Source: CAD feature listing. Evaluate the final solid. Frame: model axes, mm. Face numbers are marked on the shaded views. A direction names the side the tool comes from. Give positions to 0.01 mm unless a question says otherwise; leave off trailing zeros. Loops run counter-clockwise (first coordinate to the right, second up) from the corner with the lowest first, then second, coordinate; pieces in that order, holes last.
from build123d import *

# Parameters (mm, degrees)
F0_R     = 317.5
F1_DEPTH = 127
F2_DEPTH = 177.8
F0_R_2   = 127
F3_DEPTH = 127
F4_R     = 152.4
F5_DEPTH = 127
F6_R     = 152.4
F7_DEPTH = 127


with BuildPart() as f1:
    # F0 (on Front) → F1 (new body)
    with BuildSketch(Plane.XZ):
        with BuildLine():
            ThreePointArc((2e-06, 508), (359.210245, 359.210244), (508, 0))
            ThreePointArc((508, 0), (359.210245, -359.210244), (2e-06, -508))
            Line((2e-06, -508), (1016, -508))
            Line((1016, -508), (1016, 508))
            Line((1016, 508), (2e-06, 508))
        make_face()
        with BuildLine():
            ThreePointArc((2e-06, -508), (-508, 0), (2e-06, 508))
            Line((2e-06, 508), (-1016, 508))
            Line((-1016, 508), (-1016, -508))
            Line((-1016, -508), (2e-06, -508))
        make_face()
        with BuildLine():
            ThreePointArc((2e-06, -508), (359.210245, -359.210244), (508, 0))
            ThreePointArc((508, 0), (359.210245, 359.210244), (2e-06, 508))
            ThreePointArc((2e-06, 508), (-508, 0), (2e-06, -508))
        make_face()
        Circle(F0_R, mode=Mode.SUBTRACT)
    extrude(amount=-F1_DEPTH)

    # F0 (on Front) → F2 (join)
    with BuildSketch(Plane.XZ):
        with BuildLine():
            ThreePointArc((2e-06, -508), (359.210245, -359.210244), (508, 0))
            ThreePointArc((508, 0), (359.210245, 359.210244), (2e-06, 508))
            ThreePointArc((2e-06, 508), (-508, 0), (2e-06, -508))
        make_face()
        Circle(F0_R, mode=Mode.SUBTRACT)
    extrude(amount=F2_DEPTH)

    # F0 (on Front) → F3 (join)
    with BuildSketch(Plane.XZ):
        Circle(F0_R)
        Circle(F0_R_2, mode=Mode.SUBTRACT)
    extrude(amount=-F3_DEPTH)

    # F4 (on face) → F5 (join)
    with BuildSketch(Plane(origin=(-1016, 0, 0), x_dir=(0, -1, 0), z_dir=(-1, 0, 0))):
        with BuildLine():
            Line((-127, -508), (-127, 508))
            Line((-127, 508), (-939.8, 508))
            ThreePointArc((-939.8, 508), (-1447.8, 0), (-939.8, -508))
            Line((-939.8, -508), (-127, -508))
        make_face()
        with Locations((-939.8, 0)):
            Circle(F4_R, mode=Mode.SUBTRACT)
    extrude(amount=-F5_DEPTH)

    # F6 (on face) → F7 (join)
    with BuildSketch(Plane.YZ.offset(1016)):
        with BuildLine():
            Line((127, 508), (127, -508))
            Line((127, -508), (939.8, -508))
            ThreePointArc((939.8, -508), (1447.8, 0), (939.8, 508))
            Line((939.8, 508), (127, 508))
        make_face()
        with Locations((939.8, 0)):
            Circle(F6_R, mode=Mode.SUBTRACT)
    extrude(amount=-F7_DEPTH)


solid = f1.part
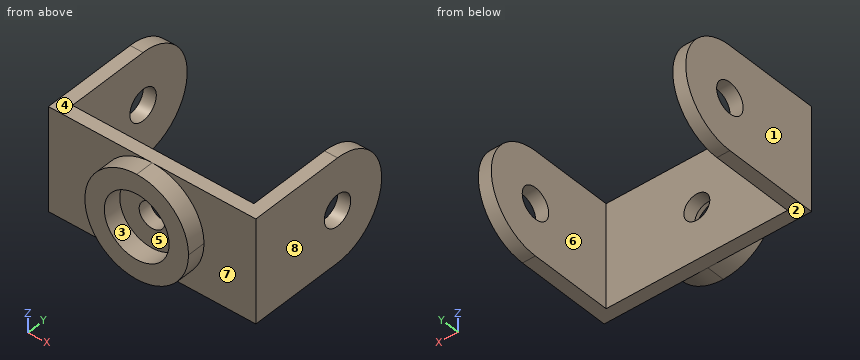
1) Ray query, probe 1 along X at (y, z) = (952, 250); probe 2 along Z at (x, y) = (-986, 939); probe 3 along Z at (x, y) = (0, 28). Return the intervals inside material, ascending.
Checks:
probe 1: x = -1016 to -889, 889 to 1016
probe 2: z = -508 to -152.4, 152.4 to 508
probe 3: z = -508 to -127, 127 to 508
2) Cut plane C-C (z = 184.5). Return loops of the section in (x, y).
Checks:
outline: (-1016, 0) - (-473.31, 0) - (-473.31, -177.8) - (-258.39, -177.8) - (-258.39, 0) - (258.39, 0) - (258.39, -177.8) - (473.31, -177.8) - (473.31, 0) - (1016, 0) - (1016, 1413.11) - (889, 1413.11) - (889, 127) - (-889, 127) - (-889, 1413.11) - (-1016, 1413.11) - close
3) Cut plane B-B (x = 419). Return loops of the section in (y, z).
Checks:
outline: (-177.8, -287.23) - (0, -287.23) - (0, -508) - (127, -508) - (127, 508) - (0, 508) - (0, 287.23) - (-177.8, 287.23) - close
4) Cut plane A-A (y = 330.5). Return loops of the section in (x, z).
Checks:
outline: (-1016, -508) - (-889, -508) - (-889, 508) - (-1016, 508) - close; (889, -508) - (1016, -508) - (1016, 508) - (889, 508) - close
5) Cut plane D-D (y = 1326.5). Return loops of the section in (x, z), and give its area (3 significant figures).
Checks:
outline: (-1016, -329.43) - (-889, -329.43) - (-889, 329.43) - (-1016, 329.43) - close; (889, -329.43) - (1016, -329.43) - (1016, 329.43) - (889, 329.43) - close
area: 167,000 mm2
6) Pull-direction query (Z, two-part tool) for the marked faces 1, 2 and 3; classes: released by +Z, released by -Z, zero draft, split by the parting line, or undercut.
Checks:
face 1: zero draft
face 2: released by -Z
face 3: undercut
7) Reachability of the marked faces 4, 5, 6, 7 and 8 from +Z, -Z, +X, -X, +Y, -Y: full face, straight path, thin tool, end or side. Return the list, or none.
Checks:
face 4: +Z, +X, -X, +Y, -Y
face 5: -Y
face 6: +Z, -Z, +Y
face 7: +X, -Y
face 8: +Z, -Z, +X, +Y, -Y
